Verification items for this drawing (mm, ordinates from the low corner). Coordinates: 2 decimals unless noted, no trailing zeros. Write each loop counter-clockwise with the first axis right and the second up, starting at its lowest first coordinate (ties: lowest second). Pieces come first, ordered by that corner, then holes. Notation, with made-up numbers: (22.25, -34.75) -> (41.25, -34.75) arc R14 ccw to (41.25, -12.75) -> close; hole circle Ø8 at (-2.5, 10.5). An arc over 180 degrees is marked (long way). One line per item, written item: value. Start each with the question number.
1) Gauge pin test, flat ends, axial feed: P1, Ø15.5, axis at x = 25.5, y = 44.5, coming from the +Z side; P2, Ø1.5, axis at y = 60.5, z = 3, coming from the +X side; P3, Ø2, axis at x = 42, z = 1, coming from the +Y side; P4, Ø2, axis at y = 27, z = 4.5, coming from the +X side (1 decimal). Record the tip position at first contact, or that the pin passes through.
2) Sectioned sample at C-C on z = 4.5. Enter the section's corners in (x, y) (1 decimal), plus the area to 3 significant figures.
3) Sectioned sample at D-D on y = 22. Enter the section's corners in (x, z).
4) Sectioned sample at B-B on y = 36.83. Enter the section's corners in (x, z), plus the area to 3 significant figures.
5) Scan lines: line 1 along Y through (x, z) = (36.83, 5.4); line 2 along Y through (x, z) = (21.5, 4.5) (1 decimal); line 3 along Y through (x, z) = (20, 4.5) (1 decimal). Record each from-to range of solid material in increasing order. Write a range as [from, to].
6) Draft check along Y on the marked faces 1, 2 and 3. Enter one of: +Y half, -Y half, draft (parallel to the pull), parting line (faces both ways), or undercut.
7) Sectioned sample at A-A on x = 36.83. Enter the section's corners in (y, z).
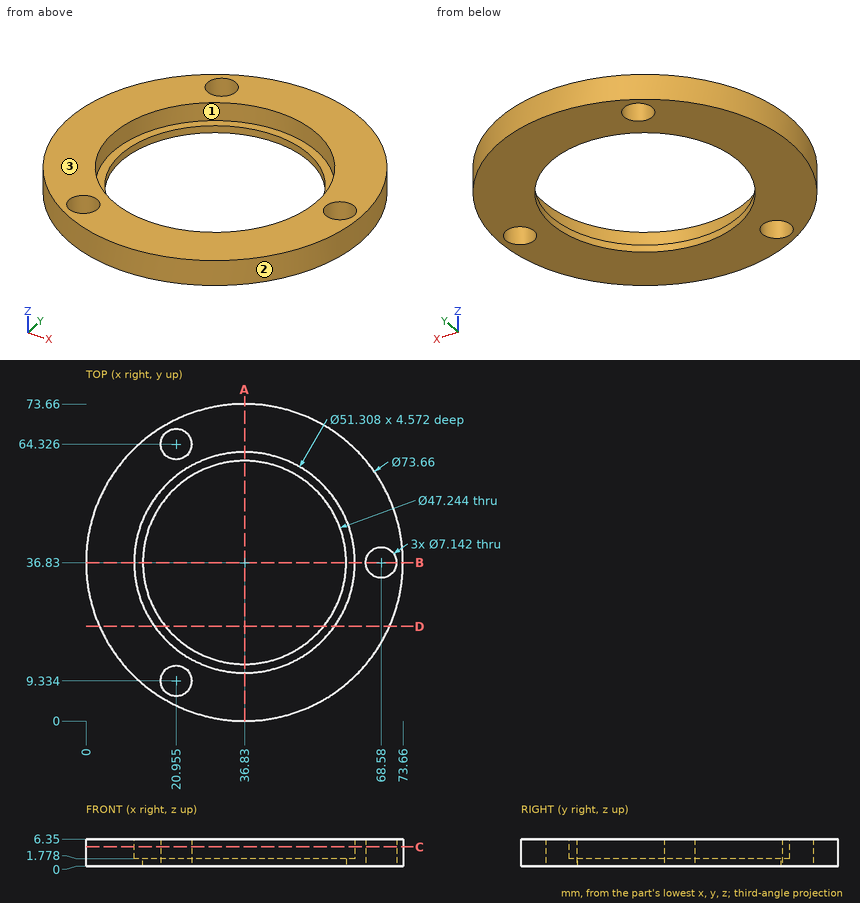
Answers:
1. P1: passes through
1. P2: stops at x = 65.66
1. P3: stops at y = 73.42
1. P4: stops at x = 72.6
2. outline: circle Ø73.7 at (36.8, 36.8); hole circle Ø51.3 at (36.8, 36.8); hole circle Ø7.1 at (21, 9.3); hole circle Ø7.1 at (21, 64.3); hole circle Ø7.1 at (68.6, 36.8)
2. area: 2,070 mm2
3. outline: (3.12, 0) -> (18.44, 0) -> (18.44, 1.78) -> (15.9, 1.78) -> (15.9, 6.35) -> (3.12, 6.35) -> close; (55.22, 0) -> (70.54, 0) -> (70.54, 6.35) -> (57.76, 6.35) -> (57.76, 1.78) -> (55.22, 1.78) -> close
4. outline: (0, 0) -> (13.21, 0) -> (13.21, 1.78) -> (11.18, 1.78) -> (11.18, 6.35) -> (0, 6.35) -> close; (60.45, 0) -> (65.01, 0) -> (65.01, 6.35) -> (62.48, 6.35) -> (62.48, 1.78) -> (60.45, 1.78) -> close; (72.15, 0) -> (73.66, 0) -> (73.66, 6.35) -> (72.15, 6.35) -> close
4. area: 104 mm2
5. line 1: y = [0, 11.18], [62.48, 73.66]
5. line 2: y = [3.3, 5.8], [12.9, 16.3], [57.4, 60.8], [67.9, 70.3]
5. line 3: y = [4.1, 5.9], [12.8, 17.5], [56.2, 60.9], [67.8, 69.6]
6. face 1: undercut
6. face 2: parting line
6. face 3: draft
7. outline: (0, 0) -> (13.21, 0) -> (13.21, 1.78) -> (11.18, 1.78) -> (11.18, 6.35) -> (0, 6.35) -> close; (60.45, 0) -> (73.66, 0) -> (73.66, 6.35) -> (62.48, 6.35) -> (62.48, 1.78) -> (60.45, 1.78) -> close
